Autodesk Inventor part; units mm, degrees
ref_plane "YZ Plane" through (0, 0, 0) normal (1, 0, 0) x (0, 1, 0)
ref_plane "XZ Plane" through (0, 0, 0) normal (0, 1, 0) x (-1, 0, 0)
ref_plane "XY Plane" through (0, 0, 0) normal (0, 0, 1) x (1, 0, 0)
sketch "Sketch1" plane through (0, 0, 0) normal (0, 1, 0) x (-1, 0, 0)
  circle A0 centre (0, 0) radius 5.4
  dimension "d0" = 10.8
extrude "Extrusion1" add sketch "Sketch1" along normal blind 73.6
sketch "Sketch2" plane through (0, 0, 0) normal (0, -1, 0) x (1, 0, 0)
  circle A0 centre (0, 0) radius 3.2
  dimension "d3" = 6.4
extrude "Extrusion2" cut sketch "Sketch2" against normal blind 70.8
sketch "Sketch3" plane through (0, 73.6, 0) normal (0, 1, 0) x (1, 0, 0)
  circle A0 centre (0, 0) radius 1.9
extrude "Extrusion3" add sketch "Sketch3" along normal blind 1
sketch "Sketch4" plane through (0, 0, 0) normal (0, -1, 0) x (1, 0, 0)
  line L0 (0, 0) -> (0, 6.725)
  line L1 (0, 6.725) -> (0, -6.725)
  line L2 (0, 6.725) -> (11.425, 6.725)
  line L3 (11.425, 6.725) -> (-11.425, 6.725)
  line L4 (-11.425, 6.725) -> (-11.425, -2.725)
  line L5 (11.425, -2.725) -> (11.425, 6.725)
  circle A0 centre (0, 0) radius 3.2
  line L6 (-11.425, 6.725) -> (-11.425, -6.725)
  line L7 (-11.425, -6.725) -> (11.425, -6.725)
  line L8 (11.425, -6.725) -> (11.425, 6.725)
  dimension "d8" = 6.725
  dimension "d9" = 13.45
  dimension "d10" = 11.425
  dimension "d11" = 22.85
  dimension "d17" = 13.45
extrude "Extrusion4" add sketch "Sketch4" along normal blind 1.75 contours A0 L1 L7 L6 L4 L3 L0 | L0 L2 L5 L8 L7 L1 A0
properties part number "SyringeBody"
CAD build for the part. Positions are in the model's coordinates, mm. A direction names the side the tool comes from. Round coordinates to 2 decimals unless told otherwise and drop trailing zeros. Order: outer loops, then holes, each group sorted by start corner. A loop starts at its lowest first (then second) coordinate and runs counter-clockwise, first axis right, second up. Notation, with made-up numbers: (29.5, -30) - (51.5, -30) arc R12 cw to (51.5, -16) - close; hole circle Ø11 at (17.25, -34.5). An arc over 180 degrees is marked (long way). Answer in a Markdown table with one row per item. Add a question column.
(1) Mould opens along Z. For faces 1 (the face through (1.17, 36.28, 5.27)), 2 (the face through (0, 70.8, 0)), 3 (the face through (0, -1, 6.725)) say: +Z half, -Z half, draft (parallel to the pull), parting line (faces both ways), or undercut.
(2) Band-saw the part on A-A on z = 0. List the corners of the cut face in (x, y) (3 decimals), and give its area (3 significant figures).
(3) 3-axis set-ups, long thin cutter, end or side, ignore diameter. For faces 4 (the face through (-1.9, 74.09, 0.08)), 5 (the face through (11.425, -1, 0)), 6 (the face through (-2.539, 35.033, 1.947)): which of +Z, -Z, +X, -X, +Y, -Y reach the whole face in a straight line?
(4) Band-saw the part on C-C on y = 68.5. List the corners of the cut face in (x, z), and give its area (3 significant figures).
(5) Drop flat-ended pins along their axis: pin 1 Ø8 at (x, y) = (2, 10) entering from -Z; pin 2 Ø6 at (y, z) = (22, -5.5) entering from -X; pin 3 Ø4 at (x, z) = (-8.5, 4) entering from +Y; pin 4 Ø7.5 at (x, z) = (0, 0) entering from -Y. Give the stop position or say it passes through.
(6) Band-saw the part on B-B on x = 0. List the corners of the cut face in (y, z) (3 decimals).
(7) Band-saw the part on D-D on z = -4.25. List the corners of the cut face in (x, y) (3 decimals), and give its area (3 significant figures).
(8) Probe L1, parallel to Z at x = 0, y = 37.5; L2, parallel to Y at x = 10.5, z = -2.5; L3, parallel to Y at x = 1.75, z = -2.75. List the from-to ranges inside material, lowest first. Write a range as [from, to].
Data:
| question | item | result |
|---|---|---|
| 1 | face 1 | parting line |
| 1 | face 2 | undercut |
| 1 | face 3 | +Z half |
| 2 | outline | (-11.425, -1.75) - (-3.2, -1.75) - (-3.2, 70.8) - (3.2, 70.8) - (3.2, -1.75) - (11.425, -1.75) - (11.425, 0) - (5.4, 0) - (5.4, 73.6) - (1.9, 73.6) - (1.9, 74.6) - (-1.9, 74.6) - (-1.9, 73.6) - (-5.4, 73.6) - (-5.4, 0) - (-11.425, 0) - close |
| 2 | area | 374 mm^2 |
| 3 | face 4 | +Y |
| 3 | face 5 | +Z, -Z, +X, +Y, -Y |
| 3 | face 6 | -Y |
| 4 | outline | circle Ø10.8 at (0, 0); hole circle Ø6.4 at (0, 0) |
| 4 | area | 59.4 mm^2 |
| 5 | pin 1 | stops at z = -5.4 |
| 5 | pin 2 | stops at x = -4.79 |
| 5 | pin 3 | stops at y = 0 |
| 5 | pin 4 | stops at y = -1.75 |
| 6 | outline | (-1.75, -6.725) - (0, -6.725) - (0, -5.4) - (73.6, -5.4) - (73.6, -1.9) - (74.6, -1.9) - (74.6, 1.9) - (73.6, 1.9) - (73.6, 5.4) - (0, 5.4) - (0, 6.725) - (-1.75, 6.725) - (-1.75, 3.2) - (70.8, 3.2) - (70.8, -3.2) - (-1.75, -3.2) - close |
| 7 | outline | (-11.425, -1.75) - (11.425, -1.75) - (11.425, 0) - (3.331, 0) - (3.331, 73.6) - (-3.331, 73.6) - (-3.331, 0) - (-11.425, 0) - close |
| 7 | area | 530 mm^2 |
| 8 | L1 | z = [-5.4, -3.2], [3.2, 5.4] |
| 8 | L2 | y = [-1.75, 0] |
| 8 | L3 | y = [-1.75, 73.6] |
